Can you work these out from the model? Positions are in its coordinate system, mm. Give positions to 0.01 mm unless a question says otherwise; leave off trailing zeros. Order: outer loops, then holes, each group sorted by start corner. A loop starts at its lowest first (then second) coordinate and runs counter-clockwise, first axis right, second up. Notation, with made-up numbers: (40, 48) - (61, 48) arc R9 cw to (61, 55) - close; hole circle Ø11 at (-20.5, 78.25). An arc over 180 degrees is marked (long way). Answer as a JSON object with one key per item and string values.
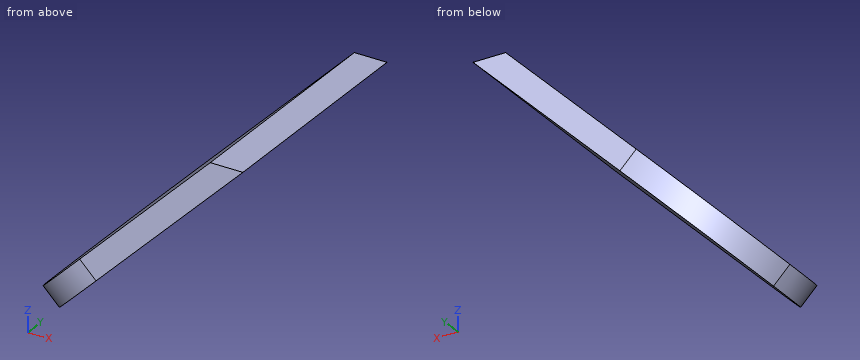
```python
from build123d import *

# Parameters (mm, degrees)
F1_DEPTH = 15.875
F3_DEPTH = 12.701


with BuildPart() as f1:
    # F0 (on Front) → F1 (new body)
    with BuildSketch(Plane.XZ):
        Polygon((2.245064, 0), (0, 0), (-14.592916, -14.592916), (-13.470384, -15.715448), align=None)
    extrude(amount=F1_DEPTH)

    # F2 (on face) → F3 (cut, through all)
    with BuildSketch(Plane(origin=(0, 0, 0), x_dir=(0, -1, 0), z_dir=(-0.707107, 0, 0.707107))):
        with BuildLine():
            ThreePointArc((7.9375, -20.6375), (2.32484, -18.31266), (0, -12.7))
            Line((0, -12.7), (0, -20.6375))
            Line((0, -20.6375), (7.9375, -20.6375))
        make_face()
        with BuildLine():
            ThreePointArc((15.875, -12.7), (13.55016, -18.31266), (7.9375, -20.6375))
            Line((7.9375, -20.6375), (15.875, -20.6375))
            Line((15.875, -20.6375), (15.875, -12.7))
        make_face()
    extrude(amount=-F3_DEPTH, mode=Mode.SUBTRACT)


solid = f1.part
```
Q1. I'm going to push flat-ended pins straight in: pin 1 Ø1.5 at (y, z) = (-13, -6) entering from +X; pin 2 Ø5 at (x, z) = (-11.5, -9.5) entering from +Y. Where does each tip first touch, or does it pass through?
Recorded:
{"pin 1": "stops at x = -3", "pin 2": "stops at y = 0"}
Q2. I need wall thicknesses on L1, parallel to Z at x = -2, y = -12.75; L2, parallel to Z at x = -1, y = -10.5; L3, parallel to X at y = -9, z = -8. Which ranges of each line are inside material? Lowest first, please.
Recorded:
{"L1": "z = -4.25 to -2", "L2": "z = -3.25 to -1", "L3": "x = -8 to -5.75"}
Q3. If we section it at B-B, the plane x = -6: Please give me the cut outline in (y, z) (3 decimals), then the cut area to 3 significant figures.
Recorded:
{"outline": "(-15.875, -8.245) - (0, -8.245) - (0, -6) - (-15.875, -6) - close", "area": "35.6 mm^2"}
Q4. If we section it at A-A, the plane y = -9.5: Please give me the cut outline in (x, z), then the cut area to 3 significant figures.
Recorded:
{"outline": "(-14.48, -14.48) - (-13.36, -15.61) - (2.25, 0) - (0, 0) - close", "area": "33.8 mm^2"}
